Geometry: final body of the model. Coordinates: model frame, mm. A direction names the side the tool comes from. Give positions to 0.01 mm unless a question says otherwise; leave off trailing zeros. Loops run counter-clockwise (first coordinate to the right, second up) from the corner with the lowest first, then second, coordinate; pieces in that order, holes last. Notation, with made-up numbers: (87.25, 1.25) -> (143.25, 1.25) arc R7 ccw to (143.25, 10.25) -> close; hole circle Ø10 at (-35, 19.5). An arc over 180 degrees is marked (long way). Answer in a Markdown table with one row per item. Add a question column.
from build123d import *

# Parameters (mm, degrees)
SKETCH_W            = 11.2
SKETCH_H            = 5.3
PAD_DEPTH           = 2.5
SKETCH001_W         = 0.25
SKETCH001_H         = 1.6
PAD001_DEPTH        = 0.2
LINEARPATTERN_COUNT = 4
LINEARPATTERN_PITCH = 1
SKETCH002_W         = 0.6
SKETCH002_H         = 3.5
POCKET_DEPTH        = 29.28159
SKETCH003_W         = 5.05
SKETCH003_H         = 1
POCKET001_DEPTH     = 3


with BuildPart() as part:
    # Sketch → Pad (new body)
    with BuildSketch(Plane.XY):
        with Locations((0, -3.45)):
            Rectangle(SKETCH_W, SKETCH_H)
    extrude(amount=PAD_DEPTH)

    # Sketch001 → Pad001 (join)
    with BuildSketch(Plane.XY):
        with Locations((-1.5, 0)):
            Rectangle(SKETCH001_W, SKETCH001_H)
    pad001 = extrude(amount=PAD001_DEPTH)

    # LinearPattern: Pad001 ×4
    with Locations(*[(i * LINEARPATTERN_PITCH, 0, 0) for i in range(1, LINEARPATTERN_COUNT)]):
        add(pad001)

    # Sketch002 → Pocket (cut, through all)
    with BuildSketch(Plane.XY):
        with Locations((-5.3, -2.55)):
            Rectangle(SKETCH002_W, SKETCH002_H)
    pocket = extrude(amount=POCKET_DEPTH, mode=Mode.SUBTRACT)

    # Mirrored: Pocket across YZ
    add(pocket.mirror(Plane.YZ), mode=Mode.SUBTRACT)

    # Sketch003 (on Face3 of Mirrored) → Pocket001 (cut)
    with BuildSketch(Plane.XZ.offset(6.1)):
        with Locations((0, 1.4)):
            Rectangle(SKETCH003_W, SKETCH003_H)
    extrude(amount=-POCKET001_DEPTH, mode=Mode.SUBTRACT)


solid = part.part
(1) Cut plane D-D on y = -2.5. Return the cut outline in (x, z).
(2) Cut plane A-A on y = 0. Return the cut outline in (x, z) (3 decimals).
(3) Pin query (flat end, axial travel): pin 1 Ø0.5 at (x, z) = (1, 1.5) entering from -Y; pin 2 Ø0.5 at (x, z) = (-5, 0.5) entering from +Y; pin 3 Ø0.7 at (x, z) = (5.5, 0.5) entering from +Y. Return the tip coordinate at first contact, or that it passes through.
(4) Cut plane B-B on z = 2.25. Return the cut outline in (x, y), then the cut area to 3 significant figures.
(5) Material intervals for line 1 along Z through (x, y) = (-2, -5.25); line 2 along X through (y, z) = (-5.5, 1) (3 decimals); line 3 along Y through (x, z) = (0, 1.85), sorted ascending. Write a range as from..to.
(6) Reachability of faces 1 (the flat face through (0, -3, 0)), 2 (the flat face through (-5, -3, 1)), 3 (the flat face through (5, -3, 1)), 4 (the flat face through (0, -3.1, 1.4)) from +Z, -Z, +X, -X, +Y, -Y: full face, straight path, thin tool, end or side. Return the list, or none.
(7) Cut plane C-C on x = 1.25. Return the cut outline in (y, z).
Answer list:
| question | item | result |
|---|---|---|
| 1 | outline | (-5, 0) -> (5, 0) -> (5, 2.5) -> (-5, 2.5) -> close |
| 2 | outline | (-1.625, 0) -> (-1.375, 0) -> (-1.375, 0.2) -> (-1.625, 0.2) -> close; (-0.625, 0) -> (-0.375, 0) -> (-0.375, 0.2) -> (-0.625, 0.2) -> close; (0.375, 0) -> (0.625, 0) -> (0.625, 0.2) -> (0.375, 0.2) -> close; (1.375, 0) -> (1.625, 0) -> (1.625, 0.2) -> (1.375, 0.2) -> close |
| 3 | pin 1 | stops at y = -3.1 |
| 3 | pin 2 | stops at y = -0.8 |
| 3 | pin 3 | stops at y = -4.3 |
| 4 | outline | (-5.6, -6.1) -> (5.6, -6.1) -> (5.6, -4.3) -> (5, -4.3) -> (5, -0.8) -> (-5, -0.8) -> (-5, -4.3) -> (-5.6, -4.3) -> close |
| 4 | area | 55.2 mm² |
| 5 | line 1 | z = 0..0.9, 1.9..2.5 |
| 5 | line 2 | x = -5.6..-2.525, 2.525..5.6 |
| 5 | line 3 | y = -3.1..-0.8 |
| 6 | face 1 | -Z, +X, -X, +Y, -Y |
| 6 | face 2 | +Z, -Z, -X, +Y |
| 6 | face 3 | +Z, -Z, +X, +Y |
| 6 | face 4 | -Y |
| 7 | outline | (-6.1, 0) -> (-0.8, 0) -> (-0.8, 2.5) -> (-6.1, 2.5) -> (-6.1, 1.9) -> (-3.1, 1.9) -> (-3.1, 0.9) -> (-6.1, 0.9) -> close |
